Autodesk Inventor part; units mm, degrees
ref_plane "YZ Plane" through (0, 0, 0) normal (1, 0, 0) x (0, 1, 0)
ref_plane "XZ Plane" through (0, 0, 0) normal (0, 1, 0) x (-1, 0, 0)
ref_plane "XY Plane" through (0, 0, 0) normal (0, 0, 1) x (1, 0, 0)
sketch "Skizze1" plane through (0, 0, 0) normal (0, 1, 0) x (-1, 0, 0)
  line L0 (0, 0) -> (32, 0)
  line L1 (32, 0) -> (32, -32)
  line L2 (32, -32) -> (0, -32)
  line L3 (0, -32) -> (0, 0)
  dimension "d0" = 32
  dimension "d1" = 32
extrude "Extrusion1" add sketch "Skizze1" along normal blind 12
sketch "Skizze2" plane through (0, 12, 0) normal (0, 1, 0) x (1, 0, 0)
  circle A0 centre (-24, 8) radius 2.2
  line L0 (-32, 32) -> (-32, 0)
  line L1 (-32, 0) -> (0, 0)
  circle A1 centre (-24, 24) radius 2.2
  circle A2 centre (-8, 8) radius 2.2
  circle A3 centre (-8, 24) radius 2.2
  dimension "d4" = 4.4
  dimension "d6" = 8
  dimension "d7" = 8
  dimension "d10" = 16
  dimension "d13" = 16
extrude "Extrusion2" cut sketch "Skizze2" against normal blind 6
chamfer "Fasen1" distance 6 angle 45 4 edges at (0, 6, 0) (-32, 6, 0) (-32, 6, -32) (0, 6, -32)
properties part number "Steckdosen_Block"
The listing builds one solid part. Answer for the finished solid, in the listing's coordinates (mm). A direction names the side the tool comes from. Coordinates: 2 decimals unless noted, no trailing zeros. Loops run counter-clockwise (first coordinate to the right, second up) from the corner with the lowest first, then second, coordinate; pieces in that order, holes last. Notation, with made-up numbers: (20.25, 29.5) -> (75.25, 29.5) arc R33 ccw to (75.25, 60.5) -> close; hole circle Ø2 at (40, 43). An arc over 180 degrees is marked (long way). Use one line per item in the form item = value. Start each with the question number.
Item 1: A tool of negligible diameter and unlimited length cuts with its end or side. For faces 5 (the face through (-24, 6, -24)), 6 (the face through (-29, 6, -3)), from which of +Z, -Z, +X, -X, +Y, -Y can it reach the whole face along a straight path? Write none if from no direction.
Item 2: The mould has two halves that part along Z. Classify faces 1 (the face through (-3, 6, -3)), 2 (the face through (-8, 6, -24)), 3 (the face through (-16, 12, -16)), 4 (the face through (-16, 6, -32)): released by +Z, released by -Z, zero draft, split by the parting line, or undercut.
Item 3: The part is cut by section A-A on y = 4.5. Determine the outline of the cut face in (x, z), then the cut area to 3 significant figures.
Item 4: Consider L1, parallel to Z at x = -24, y = 10.6; L2, parallel to Z at x = -26, y = 6.5. Determine where each line is inside the solid, lowest interval first. Write a range as [from, to].
Item 5: The part is cut by section B-B on y = 9.75. Determine the outline of the cut face in (x, z).
Item 6: The part is cut by section C-C on z = -8. Determine the outline of the cut face in (x, y), then the cut area to 3 significant figures.
Item 7: A flat-ended cylindrical pin translates along its axis: pin 1 Ø2 at (x, z) = (-8, -23) entering from +Y. Find the tip coordinate at first contact, or state that the pin passes through.
Item 8: The part is cut by section D-D on x = -24. Determine the outline of the cut face in (y, z), then the cut area to 3 significant figures.
Answer key:
q1.face_5 = +Y
q1.face_6 = +Z, -X, +Y, -Y
q2.face_1 = released by +Z
q2.face_2 = undercut
q2.face_3 = zero draft
q2.face_4 = released by -Z
q3.outline = (-32, -26) -> (-26, -32) -> (-6, -32) -> (0, -26) -> (0, -6) -> (-6, 0) -> (-26, 0) -> (-32, -6) -> close
q3.area = 952 mm2
q4.L1 = [-32, -26.2], [-21.8, -10.2], [-5.8, 0]
q4.L2 = [-32, -24.92], [-23.08, -8.92], [-7.08, 0]
q5.outline = (-32, -26) -> (-26, -32) -> (-6, -32) -> (0, -26) -> (0, -6) -> (-6, 0) -> (-26, 0) -> (-32, -6) -> close; hole circle Ø4.4 at (-24, -24); hole circle Ø4.4 at (-24, -8); hole circle Ø4.4 at (-8, -24); hole circle Ø4.4 at (-8, -8)
q6.outline = (-32, 0) -> (0, 0) -> (0, 12) -> (-5.8, 12) -> (-5.8, 6) -> (-10.2, 6) -> (-10.2, 12) -> (-21.8, 12) -> (-21.8, 6) -> (-26.2, 6) -> (-26.2, 12) -> (-32, 12) -> close
q6.area = 331 mm2
q7.pin_1 = 6
q8.outline = (0, -32) -> (12, -32) -> (12, -26.2) -> (6, -26.2) -> (6, -21.8) -> (12, -21.8) -> (12, -10.2) -> (6, -10.2) -> (6, -5.8) -> (12, -5.8) -> (12, 0) -> (0, 0) -> close
q8.area = 331 mm2
